Input: part model. Units: mm. Frame: model coordinates. Round coordinates to 2 decimals unless told otherwise and drop trailing zeros. Loops run counter-clockwise (first coordinate to the right, second up) from the corner with the lowest first, then second, coordinate; pieces in that order, holes last. Notation, with made-up numbers: M 3,-15.5 L 60,-15.5 A13 ccw 60,-0.5 Z; hole C -33.75,-33 d10. An arc over 180 degrees is marked long. Use one line per item in the form item = value. Start each with the question number.
Q1. Section query D-D, the plane x = 49.5. Output: boundary loops of the cut face in (y, z), and give its area (3 significant figures).
Q2. Ray query, line 1 along Z through (x, y) = (13, -2.1); line 2 along Z through (x, y) = (42, -1.4); line 3 along Z through (x, y) = (15, -1.4). Return the intervals inside material, ascending.
Q3. Section query B-B, the plane y = -1.75. State how many separate pieces and enclosed holes the cut face has, and give its area (3 significant figures).
Q4. Section query A-A, the plane x = 0. Output: boundary loops of the cut face in (y, z), and give its area (3 significant figures).
Q5. Mould query, pull axis Z, two halves, no side actions, for faces 1 (the cylindrical face through (34.231, -1.479, 65.813)), 2 (the cylindrical face through (26.04, -1.48, 21.63)), 3 (the flat face through (15, 0, -1)). Classes: pulls with the +Z half, pulls with the -Z half, needs draft (parallel to the pull), parting line crosses it, or undercut.
Q6. Section query C-C, the plane z = -63. Output: boundary loops of the cut face in (x, y), and give its area (3 significant figures).
```python
from build123d import *

# Parameters (mm, degrees)
SKETCH1_R           = 74.18267629
BOSS_EXTRUDE2_DEPTH = 3
SKETCH1_4_R         = 17.5
CUT_EXTRUDE1_DEPTH  = 4
SKETCH1_5_R         = 2.5
CUT_EXTRUDE2_DEPTH  = 4
SKETCH1_10_R        = 2.5
CUT_EXTRUDE5_DEPTH  = 10


with BuildPart() as part:
    # Sketch1 → Boss-Extrude2 (new body)
    with BuildSketch(Plane(origin=(0, 0, 0), x_dir=(1, 0, 0), z_dir=(0, 1, 0))):
        Circle(SKETCH1_R)
    extrude(amount=-BOSS_EXTRUDE2_DEPTH)

    # Sketch1<4> → Cut-Extrude1 (cut)
    with BuildSketch(Plane(origin=(0, 0, 0), x_dir=(1, 0, 0), z_dir=(0, 1, 0))):
        with Locations((0, 48.18267629)):
            Circle(SKETCH1_4_R)
        with Locations((45.824448258, 14.889265808)):
            Circle(SKETCH1_4_R)
        with Locations((28.321066539, -38.980603953)):
            Circle(SKETCH1_4_R)
        with Locations((-28.321066539, -38.980603953)):
            Circle(SKETCH1_4_R)
        with Locations((-45.824448258, 14.889265808)):
            Circle(SKETCH1_4_R)
    extrude(amount=-CUT_EXTRUDE1_DEPTH, mode=Mode.SUBTRACT)

    # Sketch1<5> → Cut-Extrude2 (cut)
    with BuildSketch(Plane(origin=(0, 0, 0), x_dir=(1, 0, 0), z_dir=(0, 1, 0))):
        with Locations((40.958449464, 56.374469332)):
            Circle(SKETCH1_5_R)
        with Locations((66.272163358, -21.533131187)):
            Circle(SKETCH1_5_R)
        with Locations((0, -69.68267629)):
            Circle(SKETCH1_5_R)
        with Locations((-66.605033139, -21.641287135)):
            Circle(SKETCH1_5_R)
        with Locations((-40.958449464, 56.374469332)):
            Circle(SKETCH1_5_R)
    extrude(amount=-CUT_EXTRUDE2_DEPTH, mode=Mode.SUBTRACT)

    # Sketch1<10> → Cut-Extrude5 (cut)
    with BuildSketch(Plane(origin=(0, 0, 0), x_dir=(1, 0, 0), z_dir=(0, 1, 0))):
        Circle(SKETCH1_10_R)
    extrude(amount=-CUT_EXTRUDE5_DEPTH, mode=Mode.SUBTRACT)


solid = part.part
```
Results found:
q1.outline = M -3,-55.25 L 0,-55.25 L 0,-32 L -3,-32 Z; M -3,2.22 L 0,2.22 L 0,55.25 L -3,55.25 Z
q1.area = 229 mm²
q2.line_1 = -73.03 to -59.9, -36.47 to 30.52, 47.44 to 73.03
q2.line_2 = -61.15 to -58.65, -54.1 to -31.97, 2.19 to 28.07, 49.9 to 61.15
q2.line_3 = -72.65 to -57.2, -39.17 to 27.63, 50.33 to 72.65
q3.separate_pieces = 1
q3.enclosed_holes = 11
q3.area = 12,400 mm²
q4.outline = M -3,-74.18 L 0,-74.18 L 0,-65.68 L -3,-65.68 Z; M -3,-30.68 L 0,-30.68 L 0,-2.5 L -3,-2.5 Z; M -3,2.5 L 0,2.5 L 0,67.18 L -3,67.18 Z; M -3,72.18 L 0,72.18 L 0,74.18 L -3,74.18 Z
q4.area = 310 mm²
q5.face_1 = parting line crosses it
q5.face_2 = undercut
q5.face_3 = needs draft
q6.outline = M -39.17,-3 L -9.31,-3 L -9.31,0 L -39.17,0 Z; M 9.31,-3 L 39.17,-3 L 39.17,0 L 9.31,0 Z
q6.area = 179 mm²
